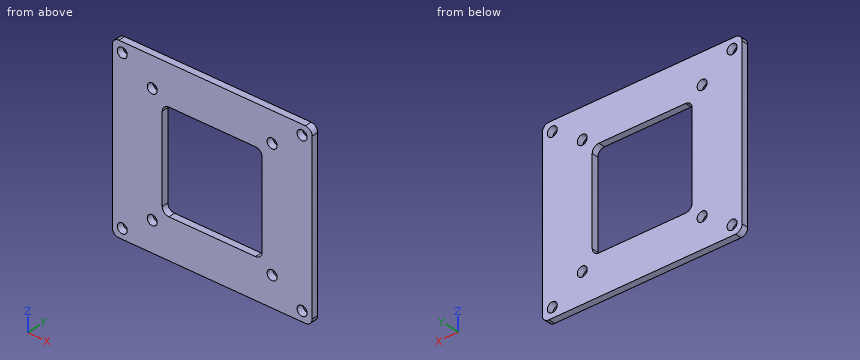
from build123d import *

# Parameters (mm, degrees)
SKETCH_1_W          = 60
SKETCH_1_H          = 54
SKETCH_1_R          = 1.5
EXTRUDE_1_DEPTH     = 2
SKETCH_2_R          = 1.5
CUT_EXTRUDE_1_DEPTH = 2
FILLET_1_R          = 2
SKETCH_3_W          = 30
SKETCH_3_H          = 30
CUT_EXTRUDE_2_DEPTH = 2
FILLET_2_R          = 2


with BuildPart() as part:
    # 草图1 → 凸台-拉伸1 (new body)
    with BuildSketch(Plane(origin=(0, 0, 0), x_dir=(1, 0, 0), z_dir=(0, 1, 0))):
        Rectangle(SKETCH_1_W, SKETCH_1_H)
        with Locations(Location((27, 24, 0), (0, 0, 270))):
            Circle(SKETCH_1_R, mode=Mode.SUBTRACT)
        with Locations(Location((-27, 24, 0), (0, 0, 90))):
            Circle(SKETCH_1_R, mode=Mode.SUBTRACT)
        with Locations(Location((-27, -24, 0), (0, 0, 270))):
            Circle(SKETCH_1_R, mode=Mode.SUBTRACT)
        with Locations(Location((27, -24, 0), (0, 0, 90))):
            Circle(SKETCH_1_R, mode=Mode.SUBTRACT)
    extrude(amount=EXTRUDE_1_DEPTH)

    # 草图2 → 切除-拉伸1 (cut)
    with BuildSketch(Plane(origin=(0, 2, 0), x_dir=(1, 0, 0), z_dir=(0, 1, 0))):
        with Locations(Location((18, 18, 0), (0, 0, 270))):
            Circle(SKETCH_2_R)
        with Locations(Location((-18, 18, 0), (0, 0, 90))):
            Circle(SKETCH_2_R)
        with Locations(Location((18, -18, 0), (0, 0, 90))):
            Circle(SKETCH_2_R)
        with Locations(Location((-18, -18, 0), (0, 0, 270))):
            Circle(SKETCH_2_R)
    extrude(amount=-CUT_EXTRUDE_1_DEPTH, mode=Mode.SUBTRACT)

    # 圆角1
    fillet_1_edges = [part.edges().sort_by_distance(p)[0] for p in [
        (30, 1, 27),
        (-30, 1, 27),
        (-30, 1, -27),
        (30, 1, -27),
    ]]
    fillet(fillet_1_edges, radius=FILLET_1_R)

    # 草图3 → 切除-拉伸2 (cut)
    with BuildSketch(Plane(origin=(0, 2, 0), x_dir=(1, 0, 0), z_dir=(0, 1, 0))):
        Rectangle(SKETCH_3_W, SKETCH_3_H)
    extrude(amount=-CUT_EXTRUDE_2_DEPTH, mode=Mode.SUBTRACT)

    # 圆角2
    fillet_2_edges = [part.edges().sort_by_distance(p)[0] for p in [
        (15, 1, -15),
        (15, 1, 15),
        (-15, 1, 15),
        (-15, 1, -15),
    ]]
    fillet(fillet_2_edges, radius=FILLET_2_R)


solid = part.part
Source: CAD feature listing. Evaluate the final solid. Frame: model axes, mm. Round coordinates to 2 decimals unless told otherwise and drop trailing zeros. Loops run counter-clockwise (first coordinate to the right, second up) from the corner with the lowest first, then second, coordinate; pieces in that order, holes last.
Q1. Ray query, line 1 (X direction, y = 1.25, z = 18); line 2 (X direction, y = 1.15, z = -24); line 3 (X direction, y = 1.7, z = 7). Return the intervals inside material, ascending.
Q2. First-contact query: P1, Ø2.5, axis at x = -18, z = -18, coming from the +Y side. Flat tip, straight axial feed; report the tip coordinate or a pass-through.
Q3. Section A-A, the plane y = 1.55. State how many separate pieces and enclosed holes the cut face has, plus the area to 3 significant figures.
Q4. Section C-C, the plane z = 9. Return loops of the section in (x, y).
Q5. Section D-D, the plane x = -6.5. Return loops of the section in (y, z), plus the area to 3 significant figures.
Q6. Section B-B, the plane x = -27. Return loops of the section in (y, z), plus the area to 3 significant figures.
Solutions:
1. line 1: x = -30 to -19.5, -16.5 to 16.5, 19.5 to 30
1. line 2: x = -30 to -28.5, -25.5 to 25.5, 28.5 to 30
1. line 3: x = -30 to -15, 15 to 30
2. P1: passes through
3. separate pieces: 1
3. enclosed holes: 9
3. area: 2,280 mm2
4. outline: (-30, 0) - (-15, 0) - (-15, 2) - (-30, 2) - close; (15, 0) - (30, 0) - (30, 2) - (15, 2) - close
5. outline: (0, -27) - (2, -27) - (2, -15) - (0, -15) - close; (0, 15) - (2, 15) - (2, 27) - (0, 27) - close
5. area: 48.0 mm2
6. outline: (0, -27) - (2, -27) - (2, -25.5) - (0, -25.5) - close; (0, -22.5) - (2, -22.5) - (2, 22.5) - (0, 22.5) - close; (0, 25.5) - (2, 25.5) - (2, 27) - (0, 27) - close
6. area: 96.0 mm2
